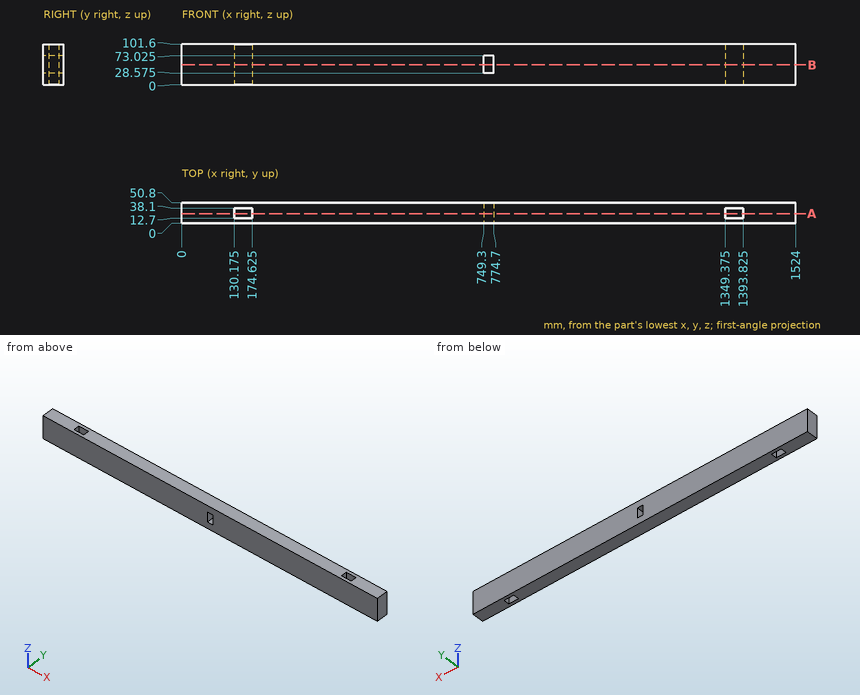
Check sheet for the drawn part. Datum: minimum x, y, z corner. Units: mm. Give positions to 0.01 mm unless a question says otherwise; leave off trailing zeros. Loops run counter-clockwise (first coordinate to the right, second up) from the corner with the lowest first, then second, coordinate; pieces in that order, holes last. Notation, with made-up numbers: (13, 37) - (34, 37) arc R29 ccw to (34, 57) - close; hole circle Ø6 at (-30, 37.5). An arc over 180 degrees is marked (long way). Write each question's results on one line, items separated by ' | '.
1) Sectioned sample at B-B on z = 50. Record the boundary of the cut face in (x, y) (3 decimals).
Solution:
outline: (0, 0) - (749.3, 0) - (749.3, 50.8) - (0, 50.8) - close; (774.7, 0) - (1524, 0) - (1524, 50.8) - (774.7, 50.8) - close; hole (130.175, 12.7) - (174.625, 12.7) - (174.625, 38.1) - (130.175, 38.1) - close; hole (1349.375, 12.7) - (1393.825, 12.7) - (1393.825, 38.1) - (1349.375, 38.1) - close
2) Depth check by flat-ended pin: P1, Ø10, axis at x = 286, z = 18, coming from the -Y side. Enter the tip coordinate at first touch or a pass-through.
Solution:
P1: y = 0
3) Sectioned sample at A-A on y = 24. Record the boundary of the cut face in (x, z) (3 decimals).
Solution:
outline: (0, 0) - (130.175, 0) - (130.175, 101.6) - (0, 101.6) - close; (174.625, 0) - (1349.375, 0) - (1349.375, 101.6) - (174.625, 101.6) - close; (1393.825, 0) - (1524, 0) - (1524, 101.6) - (1393.825, 101.6) - close; hole (749.3, 28.575) - (774.7, 28.575) - (774.7, 73.025) - (749.3, 73.025) - close
4) Material ranges on L1, parallel to X at y = 25, z = 6.5 (3 decimals); L2, parallel to X at y = 20.5, z = 29.5 (3 decimals); L3, parallel to X at y = 41.5, z = 60, recorded low to high. Write a range as from..to.
Solution:
L1: 0..130.175, 174.625..1349.375, 1393.825..1524 | L2: 0..130.175, 174.625..749.3, 774.7..1349.375, 1393.825..1524 | L3: 0..749.3, 774.7..1524
